Source: CAD feature listing. Evaluate the final solid. Frame: model axes, mm. Face numbers are marked on the shaded views. A direction names the side the tool comes from. Round coordinates to 2 decimals unless told otherwise and drop trailing zeros. Order: outer loops, then holes, each group sorted by start corner. A loop starts at its lowest first (then second) coordinate and runs counter-clockwise, first axis right, second up. Notation, with made-up numbers: M 87,25.5 L 144,25.5 A21 ccw 144,32.5 Z; hole C -2.75,35 d3. An arc over 180 degrees is marked long. Answer as CSV lines item,"result". Start each with the question number.
Item 1: Section query A-A on z = 0.95. Return the cut outline in (x, y).
Item 2: Pull-direction query (X, two-part tool) for the marked faces 1, 2 and 3; classes: +X half, -X half, draft (parallel to the pull), parting line (faces both ways), or undercut.
Item 3: Set-up query: the marked faces 4, 5 and 6. Return all of +Z, -Z, +X, -X, +Y, -Y with unobstructed straight access to the full face (end or side cutting, diameter ignored); none if empty.
Item 4: Section query C-C on z = 2.5. Return the cut outline in (x, y), plus the area to 3 significant figures.
Item 5: Line query: line 1 (Y direction, x = 0, z = 0.85); line 2 (X direction, y = 3.5, z = 3.55); line 3 (Y direction, x = -0.5, z = 0.6). Output: solid intervals per line, ascending. Write a range as [from, to].
Item 6: Section query B-B on x = -2.75. Return the cut outline in (y, z).
Item 7: First-contact query: P1, Ø0.5, axis at y = 3.5, z = 3.5, coming from the +X side; P2, Ø1.5, axis at x = 2.5, y = 1, coming from the -Z side; P3, Ø4, axis at x = 0, y = 0, coming from the +Z side. Flat tips, straight axial feed; report the tip coordinate or a pass-through.
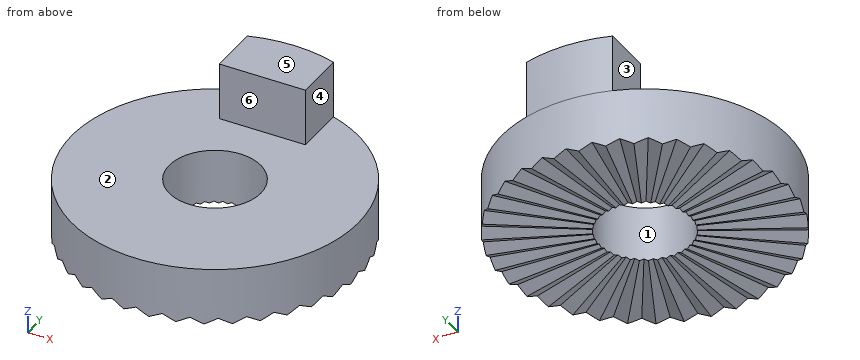
from build123d import *

# Parameters (mm, degrees)
SKETCH_1_R               = 5
SKETCH_1_R_2             = 1.6
EXTRUDE_1_DEPTH          = 2
EXTRUDE_2_DEPTH          = 2
CUT_EXTRUDE_START        = 1.574632158
CUT_EXTRUDE_1_DEPTH      = 3.428926011
PATTERN_CIRCULAR_1_COUNT = 36


# Read off the part's stored shape, not the designer's step: 切除-拉伸1
with BuildPart() as part:
    # 草图1 → 凸台-拉伸1 (new body)
    with BuildSketch(Plane.XY):
        Circle(SKETCH_1_R)
        Circle(SKETCH_1_R_2, mode=Mode.SUBTRACT)
    extrude(amount=EXTRUDE_1_DEPTH)

    # 草图2 → 凸台-拉伸2 (add)
    with BuildSketch(Plane.XY.offset(2)):
        with BuildLine():
            Line((-1.5, 4.769696007), (-1.5, 3))
            Line((-1.5, 3), (1.5, 3))
            Line((1.5, 3), (1.5, 4.769696007))
            ThreePointArc((1.5, 4.769696007), (0, 5), (-1.5, 4.769696007))
        make_face()
    extrude(amount=EXTRUDE_2_DEPTH)

    # 切除-拉伸1 outline → 切除-拉伸1 (cut)
    with BuildSketch(Plane(origin=(0, 0, 0), x_dir=(0, 1, 0), z_dir=(0.9997499284218206, 0, 0.022362482432963404)).offset(CUT_EXTRUDE_START)):
        Polygon((0.436574347, -0.111385374), (0, 0.103160358), (-0.436574347, -0.111385374), (-2, -0.879699645), (-2, -2), (2, -2), (2, -0.879699645), align=None)
    cut_extrude_1 = extrude(amount=CUT_EXTRUDE_1_DEPTH, mode=Mode.SUBTRACT)

    # 阵列(圆周)1: 切除-拉伸1 ×36 about axis
    pattern_circular_1_axis = Axis((0, 0, 0), (0, 0, 1))
    for i in range(1, PATTERN_CIRCULAR_1_COUNT):
        add(cut_extrude_1.rotate(pattern_circular_1_axis, i * 360 / PATTERN_CIRCULAR_1_COUNT), mode=Mode.SUBTRACT)


solid = part.part
Results:
1,outline,"C 0,0 d10; hole C 0,0 d3.2"
2,face 1,"undercut"
2,face 2,"draft"
2,face 3,"-X half"
3,face 4,"+Z, +X, +Y, -Y"
3,face 5,"+Z, +X, -X, +Y, -Y"
3,face 6,"+Z, +X, -X, -Y"
4,outline,"M -1.5,3 L 1.5,3 L 1.5,4.77 A5 ccw -1.5,4.77 Z"
4,area,"5.77 mm^2"
5,line 1,"[-5, -1.6], [1.6, 5]"
5,line 2,"[-1.5, 1.5]"
5,line 3,"[-4.97, -1.52], [1.52, 4.97]"
6,outline,"M -4.18,0.07 L -3.93,0 L -3.28,0.2 L -2.75,0.02 L -2.31,0.18 L -1.93,0.03 L -1.59,0.17 L -1.28,0.04 L -1,0.17 L -0.74,0.04 L -0.48,0.17 L -0.24,0.05 L 0,0.16 L 0.24,0.05 L 0.48,0.17 L 0.74,0.04 L 1,0.17 L 1.28,0.04 L 1.59,0.17 L 1.93,0.03 L 2.31,0.18 L 2.75,0.02 L 3.28,0.2 L 3.93,0 L 4.18,0.07 L 4.18,2 L -4.18,2 Z"
7,P1,"x = 1.5"
7,P2,"z = 0.03"
7,P3,"z = 2"
